CAD build for the part. Positions are in the model's coordinates, mm. Give positions to 0.01 mm unless a question says otherwise; leave off trailing zeros. Order: outer loops, then holes, each group sorted by start corner. A loop starts at its lowest first (then second) coordinate and runs counter-clockwise, first axis right, second up. Notation, with made-up numbers: M 16,65 L 50,65 A16 ccw 50,78 Z; hole C 2,0.25 d5. An arc over 180 degrees is marked long. Put each result on its own line as item: value. Start each with the question number.
1) Pin check, flat tips, straight feed: pin 1 (2 mm diameter, centred on y = -10, z = 4.5, fed in from +X); pin 2 (10 mm diameter, centred on x = 20, y = -14, fed in from -Z); pin 3 (1.5 mm diameter, centred on x = -31, z = 5.5, fed in from +Y). Stop position of each tip, or through.
2) Two-plate mould, pull along Y, no slides. Class faces 1 (the face through (11.43, -26.85, 3.76)), 2 (the face through (-12, -3, 7.62)), 3 (the face through (-26.85, -11.43, 3.76)): released by +Y, released by -Y, zero draft, split by the parting line, or undercut.
3) Cut at C-C (x = 1). Write the cut outline in (y, z), and give its area (3 significant figures).
4) Cut at A-A (z = 6). Write the cut outline in (x, y), and give its area (3 significant figures).
5) Cut at B-B (x = -22.5). Write the cut outline in (y, z), and give its area (3 significant figures).
6) Drill centre lines: line 1 (Y direction, x = 0, z = 4.25); line 2 (X direction, y = 9, z = 3); line 3 (Y direction, x = -1.5, z = 1.5). Where is each one in solid material? Low to high. Write a range as [from, to].
```python
from build123d import *

# Parameters (mm, degrees)
F0_R     = 11.5
F1_DEPTH = 7.62


with BuildPart() as f1:
    # F0 (on Top) → F1 (new body)
    with BuildSketch(Plane.XY):
        with BuildLine():
            Line((13.97, -4.2829137757), (13.97, -13.97))
            ThreePointArc((13.97, -13.97), (32.8918290507, -5.6562082279), (39.37, 13.97))
            ThreePointArc((39.37, 13.97), (26.67, 11.43), (13.97, 13.97))
            Line((13.97, 13.97), (13.97, 4.2829137757))
            ThreePointArc((13.97, 4.2829137757), (25.0565677101, 9.6203191582), (32.7279, 0))
            ThreePointArc((32.7279, 0), (25.0565677101, -9.6203191582), (13.97, -4.2829137757))
        make_face()
        with BuildLine():
            Line((4.2829137757, 13.97), (13.97, 13.97))
            ThreePointArc((13.97, 13.97), (5.6562082279, 32.8918290507), (-13.97, 39.37))
            ThreePointArc((-13.97, 39.37), (-11.43, 26.67), (-13.97, 13.97))
            Line((-13.97, 13.97), (-4.2829137757, 13.97))
            ThreePointArc((-4.2829137757, 13.97), (-5.2493849908, 31.2158008371), (9.8679, 22.86))
            ThreePointArc((9.8679, 22.86), (8.3558008371, 17.6106150092), (4.2829137757, 13.97))
        make_face()
        with BuildLine():
            ThreePointArc((-39.37, -13.97), (-26.67, -11.43), (-13.97, -13.97))
            Line((-13.97, -13.97), (-13.97, -4.2829137757))
            ThreePointArc((-13.97, -4.2829137757), (-32.7279, 0), (-13.97, 4.2829137757))
            Line((-13.97, 4.2829137757), (-13.97, 13.97))
            ThreePointArc((-13.97, 13.97), (-32.8918290507, 5.6562082279), (-39.37, -13.97))
        make_face()
        with BuildLine():
            Line((4.2829137757, -13.97), (13.97, -13.97))
            Line((13.97, -13.97), (13.97, -4.2829137757))
            ThreePointArc((13.97, -4.2829137757), (12.9921, 0), (13.97, 4.2829137757))
            Line((13.97, 4.2829137757), (13.97, 13.97))
            Line((13.97, 13.97), (4.2829137757, 13.97))
            ThreePointArc((4.2829137757, 13.97), (0, 12.9921), (-4.2829137757, 13.97))
            Line((-4.2829137757, 13.97), (-13.97, 13.97))
            Line((-13.97, 13.97), (-13.97, 4.2829137757))
            ThreePointArc((-13.97, 4.2829137757), (-13.2396808418, 2.1965677101), (-12.9921, 0))
            ThreePointArc((-12.9921, 0), (-13.2396808418, -2.1965677101), (-13.97, -4.2829137757))
            Line((-13.97, -4.2829137757), (-13.97, -13.97))
            Line((-13.97, -13.97), (-4.2829137757, -13.97))
            ThreePointArc((-4.2829137757, -13.97), (0, -12.9921), (4.2829137757, -13.97))
        make_face()
        Circle(F0_R, mode=Mode.SUBTRACT)
        with BuildLine():
            ThreePointArc((13.97, -39.37), (11.43, -26.67), (13.97, -13.97))
            Line((13.97, -13.97), (4.2829137757, -13.97))
            ThreePointArc((4.2829137757, -13.97), (8.3558008371, -17.6106150092), (9.8679, -22.86))
            ThreePointArc((9.8679, -22.86), (-5.2493849908, -31.2158008371), (-4.2829137757, -13.97))
            Line((-4.2829137757, -13.97), (-13.97, -13.97))
            ThreePointArc((-13.97, -13.97), (-5.6562082279, -32.8918290507), (13.97, -39.37))
        make_face()
    extrude(amount=F1_DEPTH)


solid = f1.part
```
Solution:
1. pin 1: x = 29.19
1. pin 2: z = 0
1. pin 3: y = 8.17
2. face 1: undercut
2. face 2: zero draft
2. face 3: released by -Y
3. outline: M -37.26,0 L -32.68,0 L -32.68,7.62 L -37.26,7.62 Z; M -13.04,0 L -11.46,0 L -11.46,7.62 L -13.04,7.62 Z; M 11.46,0 L 13.04,0 L 13.04,7.62 L 11.46,7.62 Z; M 32.68,0 L 36.25,0 L 36.25,7.62 L 32.68,7.62 Z
3. area: 86.3 mm²
4. outline: M -39.37,-13.97 A33.02 cw -13.97,-13.97 A25.4 ccw 13.97,-39.37 A33.02 cw 13.97,-13.97 A25.4 ccw 39.37,13.97 A33.02 cw 13.97,13.97 A25.4 ccw -13.97,39.37 A33.02 cw -13.97,13.97 A25.4 ccw Z; hole C -22.86,0 d19.74; hole C 0,0 d23; hole C 0,-22.86 d19.74; hole C 0,22.86 d19.74; hole C 22.86,0 d19.74
4. area: 1,270 mm²
5. outline: M -11.69,0 L -9.86,0 L -9.86,7.62 L -11.69,7.62 Z; M 9.86,0 L 12.54,0 L 12.54,7.62 L 9.86,7.62 Z
5. area: 34.4 mm²
6. line 1: [-36.78, -32.73], [-12.99, -11.5], [11.5, 12.99], [32.73, 36.78]
6. line 2: [-29.19, -26.91], [-18.81, -7.16], [7.16, 18.81], [26.91, 39.38]
6. line 3: [-35.96, -32.61], [-13.11, -11.4], [11.4, 13.11], [32.61, 37.48]
